Can you work these out from the model? Positions are in its coordinate system, mm. A direction names the side the tool comes from. Coordinates: 2 decimals unless noted, no trailing zeros. Order: outer loops, then holes, each group sorted by start corner. A loop starts at its lowest first (then second) coordinate and runs counter-clockwise, first axis right, second up. Notation, with made-up numbers: M 77,15.5 L 110,15.5 A17 cw 110,48.5 Z; hole C -13,33 d1. An arc over 180 degrees is marked long. Answer as a JSON object with one key per item and string values.
from build123d import *

# Parameters (mm, degrees)
F1_DEPTH  = 2
F2_R      = 0.35
F3_DEPTH  = 25
F4_W      = 1
F4_H      = 1.0295459899
F4_H_2    = 1.2896113173
F4_H_3    = 0.8533134981
F4_H_4    = 0.8275291947
F5_DEPTH  = 0.1
F6_W      = 1
F6_H      = 0.3036903766
F6_H_2    = 0.2311002463
F7_DEPTH  = 0.05
F9_DEPTH  = 0.1
F11_DEPTH = 0.4
F13_DEPTH = 0.15
F15_DEPTH = 0.08
F17_DEPTH = 0.08


with BuildPart() as f1:
    # F0 (on Right) → F1 (new body)
    with BuildSketch(Plane.YZ):
        Polygon((1.5289138055, 22.8420257282), (-1.5289138055, 22.8420257282), (-3.0169833821, 20.8331332634), (-1.3137839247, 18.3634953125), (-1.3137839247, 13.3634953125), (-4.8581478186, 13.3634953125), (-6.6966588007, 11.1467856193), (-5.026220344, 9.7613450914), (-3.7333500412, 11.3201707717), (-1.3137839247, 11.3201707717), (-1.3137839247, 3.3201707717), (0, 1.8122013425), (1.3137839247, 3.3201707717), (1.3137839247, 11.3201707717), (3.7333500412, 11.3201707717), (5.026220344, 9.7613450914), (6.6966588007, 11.1467856193), (4.8581478186, 13.3634953125), (1.3137839247, 13.3634953125), (1.3137839247, 18.3634953125), (3.0169833821, 20.8331332634), align=None)
    extrude(amount=F1_DEPTH)

    # F2 (on face) → F3 (cut)
    with BuildSketch(Plane.YZ.offset(2)):
        with Locations((0, 22.045429796)):
            Circle(F2_R)
    extrude(amount=-F3_DEPTH, mode=Mode.SUBTRACT)

    # F4 (on face) → F5 (cut)
    with BuildSketch(Plane.YZ.offset(2)):
        with Locations((0.0044090512, 17.6678796248)):
            Rectangle(F4_W, F4_H)
        with Locations((0.0044090512, 16.5083009712)):
            Rectangle(F4_W, F4_H_2)
        with Locations((0.0044090512, 15.4368385635)):
            Rectangle(F4_W, F4_H_3)
        with Locations((0.0044090512, 14.5964172171)):
            Rectangle(F4_W, F4_H_4)
    extrude(amount=-F5_DEPTH, mode=Mode.SUBTRACT)

    # F6 (on face) → F7 (join)
    with BuildSketch(Plane.YZ.offset(1.9)):
        with Locations((0.0044090512, 16.3344978081)):
            Rectangle(F6_W, F6_H)
        with Locations((0.0044090512, 15.2363022789)):
            Rectangle(F6_W, F6_H_2)
        with Locations((0.0044090512, 17.3582183197)):
            Rectangle(F6_W, F6_H_2)
    extrude(amount=F7_DEPTH)

    # F8 (on face) → F9 (join)
    with BuildSketch(Plane.YZ.offset(2)):
        Polygon((0.6717516341, 11.9438935243), (0, 12.8511385992), (-0.6890961678, 11.9545630374), (0, 11.023893021), align=None)
        Polygon((-0.5950663771, 11.94282338), (0, 12.7464999361), (0.5950663771, 11.94282338), (0, 11.1391468239), align=None, mode=Mode.SUBTRACT)
    extrude(amount=F9_DEPTH)

    # F10 (on face) → F11 (join)
    with BuildSketch(Plane.YZ.offset(2)):
        Polygon((4.5327297412, 12.9496529698), (1.7276167603, 12.9496529698), (1.7402404919, 12.7224316821), (4.4722869851, 12.7224316821), (5.6972301676, 11.2874979167), (5.8443970047, 11.4131281152), align=None)
    extrude(amount=-F11_DEPTH)

    # F12 (on face) → F13 (join)
    with BuildSketch(Plane.YZ.offset(2)):
        Polygon((4.5460160027, 13.0201727152), (1.7085982254, 13.0201727152), (1.7085982254, 12.9053406417), (4.4910646975, 12.9053406417), (5.7453825139, 11.386025697), (5.8344381178, 11.4595483271), align=None)
    extrude(amount=-F13_DEPTH)

    # F14 (on face) → F15 (join)
    with BuildSketch(Plane.YZ.offset(2)):
        Polygon((-4.4317739084, 12.7944620326), (-1.6240546247, 12.7944620326), (-1.6240546247, 13.0023704842), (-4.5060524717, 13.0023704842), (-6.1253183521, 11.2494025379), (-5.9816107865, 11.1166558107), align=None)
        Polygon((1.6240546247, 13.0023704842), (1.6240546247, 12.7944620326), (4.4317739084, 12.7944620326), (5.9816107865, 11.1166558107), (6.1253183521, 11.2494025379), (4.5060524717, 13.0023704842), align=None)
    extrude(amount=F15_DEPTH)

    # F16 (on face) → F17 (join)
    with BuildSketch(Plane.YZ.offset(2)):
        Polygon((-1.6705167945, 11.9723323733), (-1.6705167945, 12.2044812888), (-4.411512593, 12.2358226389), (-5.5567457362, 10.8810874), (-5.3931535222, 10.742793791), (-4.353756085, 11.9723323733), align=None)
        Polygon((4.411512593, 12.2358226389), (1.6705167945, 12.2044812888), (1.6705167945, 11.9723323733), (4.353756085, 11.9723323733), (5.3931535222, 10.742793791), (5.5567457362, 10.8810874), align=None)
    extrude(amount=F17_DEPTH)


solid = f1.part
Item 1: I want a section at B-B, the plane x = 1.6. Write out the boundary of the cut face in (y, z), plus the area to 3 significant figures.
Answers follow:
{"outline": "M -6.7,11.15 L -5.03,9.76 L -3.73,11.32 L -1.31,11.32 L -1.31,3.32 L 0,1.81 L 1.31,3.32 L 1.31,11.32 L 3.73,11.32 L 5.03,9.76 L 6.7,11.15 L 4.86,13.36 L 1.31,13.36 L 1.31,18.36 L 3.02,20.83 L 1.53,22.84 L -1.53,22.84 L -3.02,20.83 L -1.31,18.36 L -1.31,13.36 L -4.86,13.36 Z; hole C 0,22.05 d0.7", "area": "83.8 mm^2"}
Item 2: I'm going to push a flat-ended pin straight in: pin 1 (1.5 mm diameter, centred on y = 4.5, z = 20.5, fed in from -X). Where does the tip first touch, or does it pass through?
Answers follow:
{"pin 1": "passes through"}
Item 3: Please list where these lines run through material, in increasing order: line 1 (Y direction, x = 1.7, z = 5); line 2 (Z direction, x = 1.1, y = -3.5); line 3 (X direction, y = 1.25, z = 9).
Answers follow:
{"line 1": "y = -1.31 to 1.31", "line 2": "z = 11.32 to 13.36", "line 3": "x = 0 to 2"}
Item 4: I want a section at C-C, the plane y = 4. Write out the boundary of the cut face in (x, z), plus the area to 3 significant figures.
Answers follow:
{"outline": "M 0,11 L 2,11 L 2,11.97 L 2.08,11.97 L 2.08,12.23 L 2,12.23 L 2,12.79 L 2.08,12.79 L 2.08,13 L 2,13 L 2,13.36 L 0,13.36 Z", "area": "4.77 mm^2"}
Item 5: I want a section at A-A, the plane y = 2.25. Write out the boundary of the cut face in (x, z).
Answers follow:
{"outline": "M 0,11.32 L 2,11.32 L 2,11.97 L 2.08,11.97 L 2.08,12.21 L 2,12.21 L 2,12.79 L 2.08,12.79 L 2.08,13 L 2,13 L 2,13.36 L 0,13.36 Z; M 0,19.72 L 2,19.72 L 2,21.87 L 0,21.87 Z"}
Item 6: Which directions (+Z, -Z, +X, -X, +Y, -Y) give clear straight access to the entire face, cutting with the end or side of a thin tool? Please do faces 5 (the flat face through (1, -1.314, 7)), 6 (the flat face through (1.9, 0, 16)), 7 (the flat face through (1, 1.314, 16)).
Answers follow:
{"face 5": "-Z, +X, -X", "face 6": "+X", "face 7": "+X, -X, +Y"}
Item 7: If we mould it in two halves opening along Y, with no side actions, what happens to faces 1 (the flat face through (0.99, -5.87, 10.46)), 2 (the flat face through (0.99, 0.65, 2.56)), 3 (the flat face through (1, 4, 11)), 4 (the flat face through (1, -4, 11))? For each: pulls with the +Y half, pulls with the -Y half, needs draft (parallel to the pull), parting line crosses it, or undercut.
Answers follow:
{"face 1": "pulls with the -Y half", "face 2": "pulls with the +Y half", "face 3": "undercut", "face 4": "undercut"}
Item 8: I want a section at D-D, the plane z = 3. Write out the boundary of the cut face in (x, y).
Answers follow:
{"outline": "M 0,-1.03 L 2,-1.03 L 2,1.03 L 0,1.03 Z"}
